Autodesk Inventor part; units mm, degrees
ref_plane "YZ Plane" through (0, 0, 0) normal (1, 0, 0) x (0, 1, 0)
ref_plane "XZ Plane" through (0, 0, 0) normal (0, 1, 0) x (-1, 0, 0)
ref_plane "XY Plane" through (0, 0, 0) normal (0, 0, 1) x (1, 0, 0)
sketch "Sketch1" plane through (0, 0, 0) normal (1, 0, 0) x (0, 1, 0)
  arc A0 (-1.8542, -1.4222) -> (-1.8542, 1.4222) centre (0, 0) ccw
  line L0 (-2.4782, 12.4968) -> (4.3758, 12.4968)
  line L1 (7.5508, 9.3218) -> (7.5508, -9.3218)
  line L2 (4.3758, -12.4968) -> (-1.8542, -12.4968)
  line L3 (-1.8542, 12.4968) -> (-2.4782, 12.4968)
  line L4 (2.3368, 0) -> (2.3368, -12.4968) construction
  line L5 (0, 0) -> (3.6666, 0) construction
  line L6 (3.6666, 0) -> (3.6666, 12.4968) construction
  line L7 (3.6666, 0) -> (3.6666, -12.4968) construction
  arc A1 (7.5508, 9.3218) -> (4.3758, 12.4968) centre (4.3758, 9.3218) ccw
  arc A2 (4.3758, -12.4968) -> (7.5508, -9.3218) centre (4.3758, -9.3218) ccw
  line L8 (-1.8542, -12.4968) -> (-1.8542, -1.4222)
  line L9 (-1.8542, 1.4222) -> (-1.8542, 12.4968)
  dimension "d0" = 4.6736
  dimension "d4" = 10.16
  dimension "d5" = 3.175
extrude "Extrusion1" add sketch "Sketch1" along normal blind 19.05
sketch "Sketch2" plane through (0, 7.5508, 9.3218) normal (0, 1, 0) x (1, 0, 0)
  line L0 (0, 18.6436) -> (0, 0) construction
  line L1 (0, 0) -> (19.05, 0) construction
  line L2 (19.05, 18.6436) -> (19.05, 0) construction
  line L3 (0, 18.6436) -> (19.05, 18.6436) construction
  line L4 (0, 9.3218) -> (19.05, 9.3218) construction
  line L5 (9.525, 9.3218) -> (9.525, 18.6436) construction
  line L6 (0, 18.6436) -> (19.05, 18.6436) construction
  line L7 (9.525, 9.3218) -> (9.525, 0) construction
  line L8 (0, 0) -> (19.05, 0) construction
  circle A0 centre (9.525, 13.9827) radius 1.778
  circle A1 centre (9.525, 4.6609) radius 1.778
  dimension "d8" = 3.556
extrude "Extrusion2" cut sketch "Sketch2" against normal blind 19.05
properties part number "axle holder"
Geometry check sheet. Reference: the model listing, model coordinates, mm. Coordinates: 2 decimals unless noted, no trailing zeros. Order: outer loops, then holes, each group sorted by start corner. A loop starts at its lowest first (then second) coordinate and runs counter-clockwise, first axis right, second up. Notation, with made-up numbers: (-25, 28) -> (-19, 28) arc R22 ccw to (-19, 52) -> close; hole circle Ø2 at (-11, 85.5). An arc over 180 degrees is marked (long way). Use a Markdown table: item, result. Add a question column.
1. Cross-section at A-A (y = 0.5). Enter the section's corners in (x, z) (3 decimals), and give its area (3 significant figures).
2. Cross-section at B-B (x = 13.25). Enter the section's corners in (y, z) (3 decimals), and give its area (3 significant figures).
3. Mould release check, pull along X, two halves, no side actions. Record for faces 1 (the face through (0, 3, 0)), 2 (the face through (10.345, 2.914, 6.238)), 3 (the face through (10.345, 2.914, -3.084)), 4 (the face through (9.39, 6.65, -11.54)): pulls with the +X half, pulls with the -X half, needs draft (parallel to the pull), parting line crosses it, or undercut.
4. Material ranges on L1, parallel to Z at x = 4, y = 0; L2, parallel to Y at x = 5.25, z = 0; L3, parallel to X at y = 6, z = 3.75, recorded low to high.
5. Cross-section at C-C (z = -4). Enter the section's corners in (x, y), and give its area (3 significant figures).
6. Cross-section at D-D (x = 10.5). Enter the section's corners in (y, z) (3 decimals), and give its area (3 significant figures).
Filled sheet:
| question | item | result |
|---|---|---|
| 1 | outline | (0, -12.497) -> (19.05, -12.497) -> (19.05, -2.283) -> (0, -2.283) -> close; (0, 2.283) -> (19.05, 2.283) -> (19.05, 12.497) -> (0, 12.497) -> close; hole circle Ø3.556 at (9.525, -4.661); hole circle Ø3.556 at (9.525, 4.661) |
| 1 | area | 369 mm2 |
| 2 | outline | (-1.854, -12.497) -> (4.376, -12.497) arc R3.175 ccw to (7.551, -9.322) -> (7.551, 9.322) arc R3.175 ccw to (4.376, 12.497) -> (-1.854, 12.497) -> (-1.854, 1.422) arc R2.337 cw (long way) to (-1.854, -1.422) -> close |
| 2 | area | 215 mm2 |
| 3 | face 1 | pulls with the -X half |
| 3 | face 2 | undercut |
| 3 | face 3 | undercut |
| 3 | face 4 | needs draft |
| 4 | L1 | -12.5 to -2.34, 2.34 to 12.5 |
| 4 | L2 | 2.34 to 7.55 |
| 4 | L3 | 0 to 8, 11.05 to 19.05 |
| 5 | outline | (0, -1.85) -> (7.87, -1.85) -> (7.87, 7.55) -> (0, 7.55) -> close; (11.18, -1.85) -> (19.05, -1.85) -> (19.05, 7.55) -> (11.18, 7.55) -> close |
| 5 | area | 148 mm2 |
| 6 | outline | (-1.854, -12.497) -> (4.376, -12.497) arc R3.175 ccw to (7.551, -9.322) -> (7.551, -6.148) -> (-1.854, -6.148) -> close; (-1.854, -3.174) -> (7.551, -3.174) -> (7.551, 3.174) -> (-1.854, 3.174) -> (-1.854, 1.422) arc R2.337 cw (long way) to (-1.854, -1.422) -> close; (-1.854, 6.148) -> (7.551, 6.148) -> (7.551, 9.322) arc R3.175 ccw to (4.376, 12.497) -> (-1.854, 12.497) -> close |
| 6 | area | 159 mm2 |
